from build123d import *

# Parameters (mm, degrees)
SKETCH1_W           = 25.4
SKETCH1_H           = 25.4
SKETCH1_W_2         = 22.225
SKETCH1_H_2         = 22.225
BOSS_EXTRUDE1_DEPTH = 533.4
SKETCH2_R           = 4.7625
CUT_EXTRUDE1_DEPTH  = 535.155417458
SKETCH3_R           = 3.175
CUT_EXTRUDE2_DEPTH  = 535.155417458


with BuildPart() as part:
    # Sketch1 → Boss-Extrude1 (new body)
    with BuildSketch(Plane(origin=(0, 0, 0), x_dir=(0, 0, -1), z_dir=(1, 0, 0))):
        Rectangle(SKETCH1_W, SKETCH1_H)
        Rectangle(SKETCH1_W_2, SKETCH1_H_2, mode=Mode.SUBTRACT)
    extrude(amount=BOSS_EXTRUDE1_DEPTH)

    # Sketch2 → Cut-Extrude1 (cut, through all)
    with BuildSketch(Plane(origin=(0, 12.7, 0), x_dir=(1, 0, 0), z_dir=(0, 1, 0))):
        with Locations(Location((101.6, 0, 0), (0, 0, 270))):
            Circle(SKETCH2_R)
        with Locations(Location((254, 0, 0), (0, 0, 270))):
            Circle(SKETCH2_R)
    extrude(amount=-CUT_EXTRUDE1_DEPTH, mode=Mode.SUBTRACT)

    # Sketch3 → Cut-Extrude2 (cut, through all)
    with BuildSketch(Plane(origin=(0, 12.7, 0), x_dir=(1, 0, 0), z_dir=(0, 1, 0))):
        with Locations(Location((508, 0, 0), (0, 0, 270))):
            Circle(SKETCH3_R)
    extrude(amount=-CUT_EXTRUDE2_DEPTH, mode=Mode.SUBTRACT)


solid = part.part
Geometry check sheet. Reference: the model listing, model coordinates, mm. A direction names the side the tool comes from. Give positions to 0.01 mm unless a question says otherwise; leave off trailing zeros. Loops run counter-clockwise (first coordinate to the right, second up) from the corner with the lowest first, then second, coordinate; pieces in that order, holes last. Notation, with made-up numbers: (-26.75, -39.75) -> (-17.75, -39.75) arc R26 cw to (-17.75, -21.75) -> close; hole circle Ø5 at (-27, -22.75). An arc over 180 degrees is marked (long way). Answer in a Markdown table with one row per item. Add a question column.
1) Cross-section at C-C on x = 364. Record the boundary of the cut face in (y, z).
2) Draft check along Y on faces 3 (the face through (263, 12.7, 0)), 4 (the face through (533.4, 0.1, 11.3)), 5 (the face through (263, 11.112, 0)). Enter one of: pulls with the +Y half, pulls with the -Y half, needs draft (parallel to the pull), parting line crosses it, or undercut.
3) Material ranges on probe 1 along X at (y, z) = (-11.7, 0) (1 decimal); probe 2 along Y at (x, z) = (507, 3.25), recorded low to high. Write a range as from..to.
4) Cross-section at B-B on x = 101.6. Record the boundary of the cut face in (y, z).
5) Set-up check for faces 1 (the face through (263, 0, 11.112)), 2 (the face through (0, 0.1, 11.3)): record each of +Z, -Z, +X, -X, +Y, -Y from which the full face is reachable in a straight line by a thin tool's end or side.
6) Cross-section at A-A on y = -6. Record the boundary of the cut face in (x, z).
Outcome:
| question | item | result |
|---|---|---|
| 1 | outline | (-12.7, -12.7) -> (12.7, -12.7) -> (12.7, 12.7) -> (-12.7, 12.7) -> close; hole (-11.11, -11.11) -> (11.11, -11.11) -> (11.11, 11.11) -> (-11.11, 11.11) -> close |
| 2 | face 3 | pulls with the +Y half |
| 2 | face 4 | needs draft |
| 2 | face 5 | undercut |
| 3 | probe 1 | x = 0..96.8, 106.4..249.2, 258.8..504.8, 511.2..533.4 |
| 3 | probe 2 | y = -12.7..-11.11, 11.11..12.7 |
| 4 | outline | (-12.7, -12.7) -> (12.7, -12.7) -> (12.7, -4.76) -> (11.11, -4.76) -> (11.11, -11.11) -> (-11.11, -11.11) -> (-11.11, -4.76) -> (-12.7, -4.76) -> close; (-12.7, 4.76) -> (-11.11, 4.76) -> (-11.11, 11.11) -> (11.11, 11.11) -> (11.11, 4.76) -> (12.7, 4.76) -> (12.7, 12.7) -> (-12.7, 12.7) -> close |
| 5 | face 1 | +X, -X |
| 5 | face 2 | +Z, -Z, -X, +Y, -Y |
| 6 | outline | (0, -12.7) -> (533.4, -12.7) -> (533.4, -11.11) -> (0, -11.11) -> close; (0, 11.11) -> (533.4, 11.11) -> (533.4, 12.7) -> (0, 12.7) -> close |
